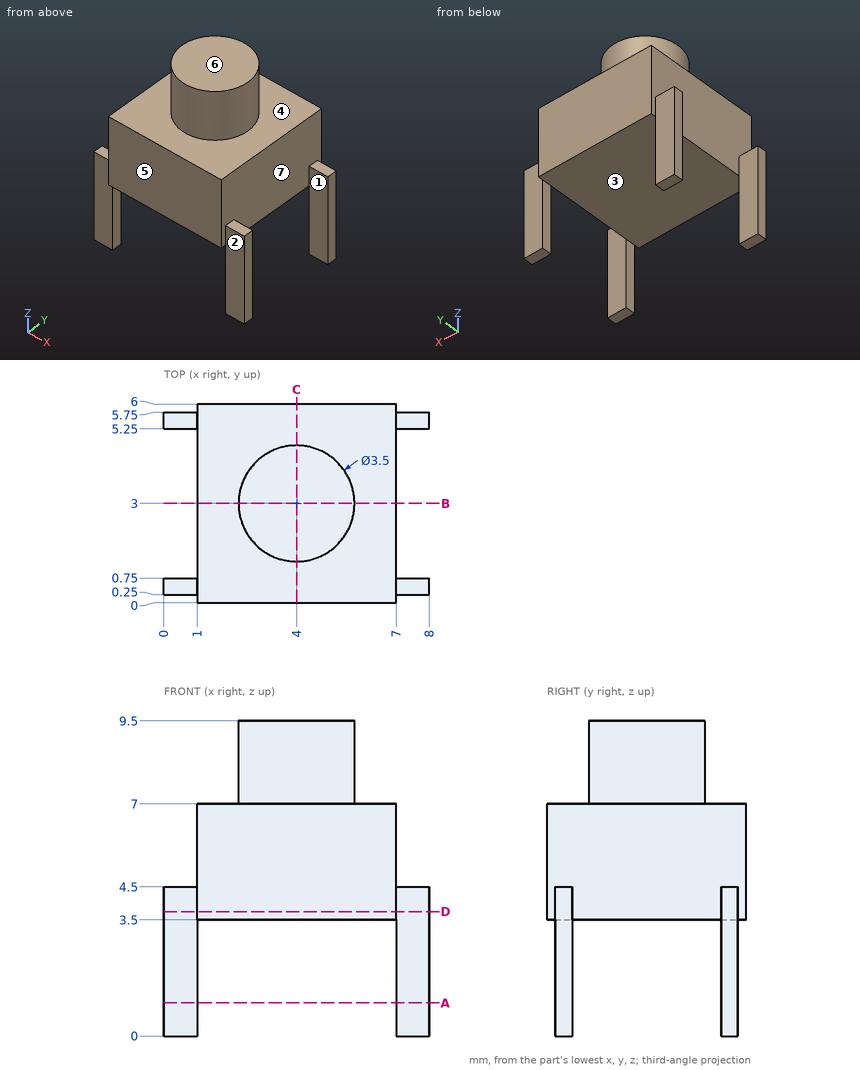
Input: dimensioned drawing with shaded views. Units: mm. Origin: part minimum x, y, z. A direction names the side the tool comes from. Give positions to 0.01 mm unless a question says otherwise; leave off trailing zeros. Order: outer loops, then holes, each group sorted by start corner. A loop starts at its lowest first (then second) coordinate and runs counter-clockwise, first axis right, second up. Notation, with made-up numbers: (-34.5, 69.25) -> (-21.5, 69.25) arc R21 ccw to (-21.5, 94.25) -> close; hole circle Ø1 at (71.5, 71.5). An arc over 180 degrees is marked (long way). Answer as a JSON object with one key per item and string values.
Q1. Section C-C (x = 4). Output: boundary loops of the cut face in (y, z), plus the area to 4 significant figures.
Entries:
{"outline": "(0, 3.5) -> (6, 3.5) -> (6, 7) -> (4.75, 7) -> (4.75, 9.5) -> (1.25, 9.5) -> (1.25, 7) -> (0, 7) -> close", "area": "29.75 mm^2"}
Q2. Material intervals for probe 1 along Z at (x, y) = (5, 1.7); probe 2 along X at (y, z) = (2.85, 6.75); probe 3 along Z at (x, y) = (2, 3.3), sorted ascending.
Entries:
{"probe 1": "z = 3.5 to 9.5", "probe 2": "x = 1 to 7", "probe 3": "z = 3.5 to 7"}
Q3. Section B-B (y = 3). Output: boundary loops of the cut face in (x, z).
Entries:
{"outline": "(1, 3.5) -> (7, 3.5) -> (7, 7) -> (5.75, 7) -> (5.75, 9.5) -> (2.25, 9.5) -> (2.25, 7) -> (1, 7) -> close"}
Q4. Access query for the marked faces 1, 2, 3 and 4. Directions: +Z, -Z, +X, -X, +Y, -Y. A direction counts if a zero-diameter tool reaches every point of the face in a straight line with its end or side. Return the directions, or none.
Entries:
{"face 1": "+Z, -Z, +X", "face 2": "+Z, -Z, +X, -Y", "face 3": "-Z, +Y, -Y", "face 4": "+Z"}
Q5. Draft query along Y for the marked faces 5, 6 and 7. Return one class per face: released by +Y, released by -Y, zero draft, split by the parting line, or undercut.
Entries:
{"face 5": "released by -Y", "face 6": "zero draft", "face 7": "undercut"}
Q6. First-contact query: pin 1 (1.8 mm diameter, centred on y = 4.5, z = 6, fed in from +X); pin 2 (0.5 mm diameter, centred on x = 7.5, z = 3, fed in from -Y); pin 3 (0.5 mm diameter, centred on x = 0.5, z = 1.5, fed in from +Y). Flat tips, straight axial feed; report the tip coordinate or a pass-through.
Entries:
{"pin 1": "stops at x = 7", "pin 2": "stops at y = 0.25", "pin 3": "stops at y = 5.75"}
Q7. Section D-D (z = 3.75). Output: boundary loops of the cut face in (x, y).
Entries:
{"outline": "(0, 0.25) -> (1, 0.25) -> (1, 0) -> (7, 0) -> (7, 0.25) -> (8, 0.25) -> (8, 0.75) -> (7, 0.75) -> (7, 5.25) -> (8, 5.25) -> (8, 5.75) -> (7, 5.75) -> (7, 6) -> (1, 6) -> (1, 5.75) -> (0, 5.75) -> (0, 5.25) -> (1, 5.25) -> (1, 0.75) -> (0, 0.75) -> close"}
Q8. Section A-A (z = 1). Output: boundary loops of the cut face in (x, y).
Entries:
{"outline": "(0, 0.25) -> (1, 0.25) -> (1, 0.75) -> (0, 0.75) -> close; (0, 5.25) -> (1, 5.25) -> (1, 5.75) -> (0, 5.75) -> close; (7, 0.25) -> (8, 0.25) -> (8, 0.75) -> (7, 0.75) -> close; (7, 5.25) -> (8, 5.25) -> (8, 5.75) -> (7, 5.75) -> close"}
